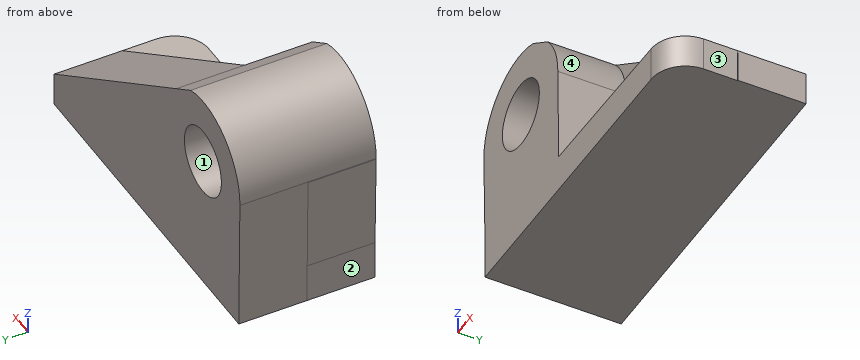
```python
from build123d import *

# Parameters (mm, degrees)
F0_R     = 12.7
F1_DEPTH = 25.4
F2_R     = 12.7
F3_DEPTH = 25.4
F4_R     = 12.7


with BuildPart() as f1:
    # F0 (on Front) → F1 (new body)
    with BuildSketch(Plane.XZ):
        with BuildLine():
            Line((22.6161210575, -50.3441899378), (-61.2315756106, 3.798879284))
            Line((-61.2315756106, 3.798879284), (-71.0548742693, 10.14208918))
            ThreePointArc((-71.0548742693, 10.14208918), (-94.3608422008, 6.8416897346), (-104.9488988238, -14.1810083481))
            Line((-104.9488988238, -14.1810083481), (-104.1759357505, -64.9751273787))
            Line((-104.1759357505, -64.9751273787), (22.8093618259, -63.0427196954))
            Line((22.8093618259, -63.0427196954), (22.6161210575, -50.3441899378))
        make_face()
        with Locations((-79.5518393085, -13.7945268115)):
            Circle(F0_R, mode=Mode.SUBTRACT)
    extrude(amount=F1_DEPTH)

    # F2 (on face) → F3 (join)
    with BuildSketch(Plane.XZ.offset(25.4)):
        with BuildLine():
            Line((-61.2315756106, 3.798879284), (-71.0548742693, 10.14208918))
            ThreePointArc((-71.0548742693, 10.14208918), (-94.3608422008, 6.8416897346), (-104.9488988238, -14.1810083481))
            Line((-104.9488988238, -14.1810083481), (-104.9422175693, -14.4935917412))
            Line((-104.9422175693, -14.4935917412), (-104.1759357505, -50.3441899378))
            Line((-104.1759357505, -50.3441899378), (-104.1759357505, -64.9751273787))
            Line((-104.1759357505, -64.9751273787), (22.6161210575, -63.0456603504))
            Line((22.6161210575, -63.0456603504), (22.6161210575, -50.3441899378))
            Line((22.6161210575, -50.3441899378), (-53.5956422432, -50.3441899378))
            Line((-53.5956422432, -50.3441899378), (-54.1518393085, -13.7945268115))
            ThreePointArc((-54.1518393085, -13.7945268115), (-55.9881522251, -4.3122986431), (-61.2315756106, 3.798879284))
        make_face()
        with Locations((-79.5518393085, -13.7945268115)):
            Circle(F2_R, mode=Mode.SUBTRACT)
    extrude(amount=F3_DEPTH)

    # F4
    f4_edges = [f1.edges().sort_by_distance(p)[0] for p in [
        (22.616121, -50.8, -56.694925),
    ]]
    fillet(f4_edges, radius=F4_R)


solid = f1.part
```
Read the model definition and answer for the solid it produces. Units are mm, in the model's axes. Face numbers are marked on the shaded views. A direction names the side the tool comes from. Give positions to 0.01 mm unless a question says otherwise; leave off trailing zeros. Loops run counter-clockwise (first coordinate to the right, second up) from the corner with the lowest first, then second, coordinate; pieces in that order, holes last.
Item 1: The part is cut by section D-D (y = -30). Write down the section's boundary in (x, z), and give its area (3 significant figures).
Item 2: For the marked faces 1, 2, 3 and 4, determine the directions among +Z, -Z, +X, -X, +Y, -Y from which every point of the face is accessible in a straight line to the end or side of a thin tool.
Item 3: Each of these flat-tipped pins is pushed along its axis until it touches: pin 1 Ø8 at (x, y) = (-87, -25.5) entering from +Z; pin 2 Ø1 at (x, z) = (-79.5, -2) entering from +Y; pin 3 Ø4 at (y, z) = (-33.5, -58.5) entering from +X; pin 4 Ø6 at (y, z) = (-35, -27.5) entering from -X. Where does it stop, or does it pass through?
Item 4: The part is cut by section B-B (x = -79). Write down the section's boundary in (y, z).
Item 5: Find the intervals of material crossed by line 1 along X through (y, z) = (-28, -51.5); line 2 along X through (y, z) = (-27, -12); line 3 along Y through (x, z) = (-34.5, -37.5), in increasing order.
Item 6: The part is cut by section A-A (y = -16). Write down the section's boundary in (x, z), and give its area (3 significant figures).
Taken from the geometry:
1. outline: (-104.95, -14.18) - (-104.18, -50.34) - (-104.18, -64.98) - (22.62, -63.05) - (22.62, -50.34) - (-53.6, -50.34) - (-54.15, -13.79) arc R25.4 ccw to (-61.23, 3.8) - (-71.05, 10.14) arc R25.4 ccw to start; hole circle Ø25.4 at (-79.55, -13.79)
1. area: 4,090 mm2
2. face 1: +Y, -Y
2. face 2: -Z, -X, -Y
2. face 3: +Z, -Z, +X, -Y
2. face 4: +Z, +X, -Y
3. pin 1: stops at z = 11.37
3. pin 2: passes through
3. pin 3: stops at x = 22.62
3. pin 4: stops at x = -104.73
4. outline: (-50.8, -64.59) - (0, -64.59) - (0, -26.48) - (-50.8, -26.48) - close; (-50.8, -1.11) - (0, -1.11) - (0, 11.6) - (-50.8, 11.6) - close
5. line 1: x = -104.18 to 22.62
5. line 2: x = -104.89 to -92.12, -66.98 to -54.22
5. line 3: y = -25.4 to 0
6. outline: (-104.95, -14.18) - (-104.18, -64.98) - (22.81, -63.04) - (22.62, -50.34) - (-71.05, 10.14) arc R25.4 ccw to start; hole circle Ø25.4 at (-79.55, -13.79)
6. area: 6,010 mm2
